```python
from build123d import *

# Parameters (mm, degrees)
SKETCH1_W                       = 114.3
SKETCH1_H                       = 177.8
SKETCH1_W_2                     = 101.6
SKETCH1_H_2                     = 165.1
BOSS_EXTRUDE1_DEPTH             = 4.7625
SKETCH2_W                       = 12.38677804
SKETCH2_H                       = 4.7625
SKETCH2_W_2                     = 12.7
BOSS_EXTRUDE2_DEPTH             = 4.7625
SKETCH3_W                       = 12.7
SKETCH3_H                       = 4.7625
BOSS_EXTRUDE3_DEPTH             = 4.7625
SKETCH4_W                       = 9.525
SKETCH4_H                       = 177.8
SKETCH4_W_2                     = 3.81
SKETCH4_H_2                     = 127
BOSS_EXTRUDE4_DEPTH             = 4.7625
FILLET1_R                       = 1.905
F_9_64_0_14063_DIAMETER_HOLE1_D = 3.572002


with BuildPart() as part:
    # Sketch1 → Boss-Extrude1 (new body)
    with BuildSketch(Plane(origin=(0, 0, 0), x_dir=(1, 0, 0), z_dir=(0, 1, 0))):
        Rectangle(SKETCH1_W, SKETCH1_H)
        Rectangle(SKETCH1_W_2, SKETCH1_H_2, mode=Mode.SUBTRACT)
    extrude(amount=BOSS_EXTRUDE1_DEPTH)

    # Sketch2 → Boss-Extrude2 (add)
    with BuildSketch(Plane.XY.offset(88.9)):
        with Locations((-38.1, 2.38125)):
            Rectangle(SKETCH2_W, SKETCH2_H)
        with Locations((12.7, 2.38125)):
            Rectangle(SKETCH2_W_2, SKETCH2_H)
    extrude(amount=BOSS_EXTRUDE2_DEPTH)

    # Sketch3 → Boss-Extrude3 (add)
    with BuildSketch(Plane(origin=(0, 0, -88.9), x_dir=(-1, 0, 0), z_dir=(0, 0, -1))):
        with Locations((-38.1, 2.38125)):
            Rectangle(SKETCH3_W, SKETCH3_H)
        with Locations((12.7, 2.38125)):
            Rectangle(SKETCH3_W, SKETCH3_H)
    extrude(amount=BOSS_EXTRUDE3_DEPTH)

    # Sketch4 → Boss-Extrude4 (add)
    # profile 1 of 2: a face of its own
    with BuildSketch(Plane(origin=(0, 4.7625, 0), x_dir=(-1, 0, 0), z_dir=(0, 1, 0))):
        with Locations((9.906, 0)):
            Rectangle(SKETCH4_W, SKETCH4_H)
        with Locations((9.906, 0)):
            Rectangle(SKETCH4_W_2, SKETCH4_H_2, mode=Mode.SUBTRACT)
    # profile 2 of 2: a face of its own
    with BuildSketch(Plane(origin=(0, 4.7625, 0), x_dir=(-1, 0, 0), z_dir=(0, 1, 0))):
        with Locations((-9.906, 0)):
            Rectangle(SKETCH4_W, SKETCH4_H)
        with Locations((-9.906, 0)):
            Rectangle(SKETCH4_W_2, SKETCH4_H_2, mode=Mode.SUBTRACT)
    extrude(amount=-BOSS_EXTRUDE4_DEPTH)

    # Fillet1
    fillet1_edges = [part.edges().sort_by_distance(p)[0] for p in [
        (-8.001, 2.38125, -63.5),
        (-11.811, 2.38125, -63.5),
        (8.001, 2.38125, -63.5),
        (11.811, 2.38125, -63.5),
        (-8.001, 2.38125, 63.5),
        (-11.811, 2.38125, 63.5),
        (8.001, 2.38125, 63.5),
        (11.811, 2.38125, 63.5),
        (-5.1435, 2.38125, 82.55),
        (5.1435, 2.38125, 82.55),
        (-5.1435, 2.38125, -82.55),
        (5.1435, 2.38125, -82.55),
        (-14.6685, 2.38125, -82.55),
        (-50.8, 2.38125, -82.55),
        (-50.8, 2.38125, 82.55),
        (-14.6685, 2.38125, 82.55),
        (14.6685, 2.38125, 82.55),
        (50.8, 2.38125, 82.55),
        (14.6685, 2.38125, -82.55),
        (50.8, 2.38125, -82.55),
    ]]
    fillet(fillet1_edges, radius=FILLET1_R - 0.0001)  # a hair under: the kernel refuses the full size

    # 9/64 (0.14063) Diameter Hole1 (through all)
    with Locations(Plane(origin=(0, 4.7625, 0), x_dir=(-1, 0, 0), z_dir=(0, 1, 0))):
        with Locations((32.73425, -85.725), (-32.73425, -85.725), (32.73425, 85.725), (-32.73425, 85.725)):
            Hole(F_9_64_0_14063_DIAMETER_HOLE1_D / 2)


solid = part.part
```
For this review, take the finished solid that the model builds, in its own axes (mm). A direction names the side the tool comes from. Round coordinates to 2 decimals unless told otherwise and drop trailing zeros. Write each loop counter-clockwise with the first axis right and the second up, starting at its lowest first coordinate (ties: lowest second). Pieces come first, ordered by that corner, then holes. Notation, with made-up numbers: (26, 17) - (79, 17) arc R18 ccw to (79, 39) - close; hole circle Ø5 at (87.25, -32). An arc over 180 degrees is marked (long way). Write each question's results on one line, items separated by ' | '.
Item 1: Draft analysis for pull direction X (two halves, no side actions). For faces 1 (the face through (-19.05, 2, -91)), 2 (the face through (14.669, 2, -1)), 3 (the face through (51, 2, -88.9)), 4 (the face through (-33, 2, 82.55)), state which applies: pulls with the +X half, pulls with the -X half, needs draft (parallel to the pull), parting line crosses it, or undercut.
Calculated:
face 1: pulls with the -X half | face 2: undercut | face 3: needs draft | face 4: undercut
Item 2: Take a section at B-B on x = 42. State the section outline as (y, z) points, then the cut area to 3 significant figures.
Calculated:
outline: (0, -93.66) - (4.76, -93.66) - (4.76, -82.55) - (0, -82.55) - close; (0, 82.55) - (4.76, 82.55) - (4.76, 88.9) - (0, 88.9) - close | area: 83.2 mm^2
Item 3: To check wall thickness, follow line 1 along X through (y, z) = (3.75, -23); line 2 along X through (y, z) = (0.45, 74); line 3 along Z through (x, y) = (44, 4.65). State the ranges of each line that lie inside material, in increasing order. Write a range as from..to.
Calculated:
line 1: x = -57.15..-50.8, -14.67..-11.81, -8..-5.14, 5.14..8, 11.81..14.67, 50.8..57.15 | line 2: x = -57.15..-50.8, -14.67..-5.14, 5.14..14.67, 50.8..57.15 | line 3: z = -93.66..-82.55, 82.55..88.9
Item 4: For pin 1 (1.4 mm diameter, centred on x = 51.5, y = 2.5, fed in from -Z); pin 2 (2.5 mm diameter, centred on y = 3.5, z = -91, fed in from +X); pin 3 (1.4 mm diameter, centred on x = -1.5, y = 3, fed in from +Z), all flat-tipped, find the tip position at first contact; note any pin that passes through.
Calculated:
pin 1: stops at z = -88.9 | pin 2: stops at x = 44.45 | pin 3: stops at z = 88.9
Item 5: Take a section at C-C on y = 1.85. Count the separate pieces of the cut face and the enclosed holes in it, then the cut area to 3 significant figures.
Calculated:
separate pieces: 1 | enclosed holes: 9 | area: 5,940 mm^2
Item 6: Take a section at A-A on z = -15.5. State the section outline as (x, y) points.
Calculated:
outline: (-57.15, 0) - (-50.8, 0) - (-50.8, 4.76) - (-57.15, 4.76) - close; (-14.67, 0) - (-11.81, 0) - (-11.81, 4.76) - (-14.67, 4.76) - close; (-8, 0) - (-5.14, 0) - (-5.14, 4.76) - (-8, 4.76) - close; (5.14, 0) - (8, 0) - (8, 4.76) - (5.14, 4.76) - close; (11.81, 0) - (14.67, 0) - (14.67, 4.76) - (11.81, 4.76) - close; (50.8, 0) - (57.15, 0) - (57.15, 4.76) - (50.8, 4.76) - close
Item 7: For faces 5 (the face through (6.35, 2, 91)), 6 (the face through (33, 2, 82.55)), 7 (the face through (38, 2, 88.9)), 8 (the face through (31.75, 2, -91)), list the 3-axis set-ups (+Z, -Z, +X, -X, +Y, -Y) from which the entire face can be reached by the end or side of a thin tool; tool diameter is ignored.
Calculated:
face 5: +Z, +Y, -Y | face 6: +Y, -Y | face 7: +Z, +X, +Y, -Y | face 8: -Z, +Y, -Y
